Source: CAD feature listing. Evaluate the final solid. Frame: model axes, mm. Face numbers are marked on the shaded views. A direction names the side the tool comes from. Give positions to 0.01 mm unless a question says otherwise; leave off trailing zeros. Order: outer loops, then holes, each group sorted by start corner. A loop starts at its lowest first (then second) coordinate and runs counter-clockwise, first axis right, second up.
```python
from build123d import *

# Parameters (mm, degrees)
SKETCH1_R           = 1.6
BOSS_EXTRUDE1_DEPTH = 10
CAVITY1_OUTLINE_R   = 1.25
CAVITY1_DEPTH       = 6.34
CAVITY1_START       = -22.606898648
CAVITY1_2_OUTLINE_R = 0.9
CAVITY1_2_DEPTH     = 0.47
CAVITY1_START_2     = -15.306898648
CAVITY1_3_OUTLINE_R = 0.9
CAVITY1_3_DEPTH     = 0.47
CAVITY1_START_3     = -6.506898648
CAVITY1_4_OUTLINE_R = 0.9
CAVITY1_4_DEPTH     = 0.47
CUT_EXTRUDE2_REACH  = 54.912
SKETCH2_R           = 1.15
CUT_EXTRUDE3_START  = -3.5
SKETCH3_R           = 1.15
CUT_EXTRUDE3_DEPTH  = 3.5
FILLET1_R           = 1
FILLET2_R           = 5
CUT_EXTRUDE4_START  = -6.34
CUT_EXTRUDE4_DEPTH  = 6.34
FILLET3_R           = 2
FILLET4_R           = 2
FILLET5_R           = 0.5


with BuildPart() as part:
    # Sketch1 → Boss-Extrude1 (new body)
    with BuildSketch(Plane.XY):
        Polygon((0, 0), (25.6, 0), (38.35, -30.037117664), (38.35, -35.9), (15.869351212, -35.9), (0, -28.5), align=None)
        with Locations((31.648794461, -31.570900751)):
            Circle(SKETCH1_R, mode=Mode.SUBTRACT)
        with Locations((21.498394042, -9.298229799)):
            Circle(SKETCH1_R, mode=Mode.SUBTRACT)
    extrude(amount=BOSS_EXTRUDE1_DEPTH)

    # Cavity1: read off the stored shape, not the designer's step
    # Cavity1 outline → Cavity1 (cut)
    with BuildSketch(Plane.XY):
        Polygon((10.198394042, -24.671898648), (10.198394042, -21.671898648), (10.808394042, -21.171898648), (10.808394042, -18.171898648), (10.198394042, -17.671898648), (10.198394042, -12.171898648), (10.808394042, -11.671898648), (10.808394042, -8.671898648), (10.198394042, -8.171898648), (10.198394042, -4.671898648), (0, -4.671898648), (0, -14.603899938), (0.718394042, -15.191898648), (0.718394042, -24.671898648), align=None)
        with Locations((7.908394042, -19.671898648)):
            Circle(CAVITY1_OUTLINE_R, mode=Mode.SUBTRACT)
        with Locations((7.908394042, -10.171898648)):
            Circle(CAVITY1_OUTLINE_R, mode=Mode.SUBTRACT)
    extrude(amount=CAVITY1_DEPTH, mode=Mode.SUBTRACT)

    # Cavity1 2 outline → Cavity1 2 (cut)
    with BuildSketch(Plane(origin=(0, 0, 0), x_dir=(1, 0, 0), z_dir=(0, 1, 0)).offset(CAVITY1_START)):
        Polygon((13.478394042, -4.73), (14.198394042, -4.01), (14.198394042, -2.33), (13.478394042, -1.61), (10.198394042, -1.61), (10.198394042, -4.73), align=None)
        with Locations((12.398394042, -3.17)):
            Circle(CAVITY1_2_OUTLINE_R, mode=Mode.SUBTRACT)
    extrude(amount=CAVITY1_2_DEPTH, mode=Mode.SUBTRACT)

    # Cavity1 3 outline → Cavity1 3 (cut)
    with BuildSketch(Plane(origin=(0, 0, 0), x_dir=(1, 0, 0), z_dir=(0, 1, 0)).offset(CAVITY1_START_2)):
        Polygon((13.478394042, -4.73), (14.198394042, -4.01), (14.198394042, -2.33), (13.478394042, -1.61), (10.198394042, -1.61), (10.198394042, -4.73), align=None)
        with Locations((12.398394042, -3.17)):
            Circle(CAVITY1_3_OUTLINE_R, mode=Mode.SUBTRACT)
    extrude(amount=CAVITY1_3_DEPTH, mode=Mode.SUBTRACT)

    # Cavity1 4 outline → Cavity1 4 (cut)
    with BuildSketch(Plane(origin=(0, 0, 0), x_dir=(1, 0, 0), z_dir=(0, 1, 0)).offset(CAVITY1_START_3)):
        Polygon((13.478394042, -4.73), (14.198394042, -4.01), (14.198394042, -2.33), (13.478394042, -1.61), (10.198394042, -1.61), (10.198394042, -4.73), align=None)
        with Locations((12.398394042, -3.17)):
            Circle(CAVITY1_4_OUTLINE_R, mode=Mode.SUBTRACT)
    extrude(amount=CAVITY1_4_DEPTH, mode=Mode.SUBTRACT)

    # Cut-Extrude2: up to this face of the body (flat: up to its plane)
    cut_extrude2_end = Plane(part.part.faces().sort_by_distance((19.850612991, -19.341556746, 0))[0])
    # Sketch2 → Cut-Extrude2 (cut, up to the picked face)
    with BuildSketch(Plane(origin=(0, 0, 6.34), x_dir=(-1, 0, 0), z_dir=(0, 0, -1)), mode=Mode.PRIVATE) as cut_extrude2_sk1:
        Polygon((-10.908394042, -21.219231953), (-10.298394042, -21.719231953), (-10.298394042, -24.771898648), (-0.618394042, -24.771898648), (-0.618394042, -15.239275241), (0.1, -14.651276531), (0.1, -4.571898648), (-10.298394042, -4.571898648), (-10.298394042, -8.124565343), (-10.908394042, -8.624565343), (-10.908394042, -11.719231953), (-10.298394042, -12.219231953), (-10.298394042, -17.624565343), (-10.908394042, -18.124565343), align=None)
        with Locations((-7.908394042, -10.171898648)):
            Circle(SKETCH2_R, mode=Mode.SUBTRACT)
        with Locations((-7.908394042, -19.671898648)):
            Circle(SKETCH2_R, mode=Mode.SUBTRACT)
    cut_extrude2_tool1 = split(extrude(cut_extrude2_sk1.sketch, amount=CUT_EXTRUDE2_REACH, mode=Mode.PRIVATE), bisect_by=cut_extrude2_end, keep=Keep.BOTH, mode=Mode.PRIVATE)
    add(cut_extrude2_tool1.solids().sort_by(Axis((5.274649, -14.483088, 6.34), (0, 0, -1)))[0], mode=Mode.SUBTRACT)

    # Sketch3 → Cut-Extrude3 (cut)
    with BuildSketch(Plane(origin=(0, 0, 0), x_dir=(-1, 0, 0), z_dir=(0, 0, -1)).offset(CUT_EXTRUDE3_START)):
        with Locations((-7.908394042, -10.171898648)):
            Circle(SKETCH3_R)
        with Locations((-7.908394042, -19.671898648)):
            Circle(SKETCH3_R)
    extrude(amount=CUT_EXTRUDE3_DEPTH, mode=Mode.SUBTRACT)

    # Fillet1
    fillet1_edges = [part.edges().sort_by_distance(p)[0] for p in [
        (9.058394042, -10.171898648, 3.5),
        (9.058394042, -19.671898648, 3.5),
    ]]
    fillet(fillet1_edges, radius=FILLET1_R)

    # Fillet2
    fillet2_edges = [part.edges().sort_by_distance(p)[0] for p in [
        (25.6, 0, 5),
        (38.35, -30.037117664, 5),
    ]]
    fillet(fillet2_edges, radius=FILLET2_R)

    # Sketch4 → Cut-Extrude4 (cut)
    with BuildSketch(Plane(origin=(0, 0, 0), x_dir=(-1, 0, 0), z_dir=(0, 0, -1)).offset(CUT_EXTRUDE4_START)):
        Polygon((-10.298394042, -5.850997484), (-15.298394042, -5.850997484), (-23.35, -35.9), (-17.655981008, -35.9), (-14.377222224, -23.663505632), (-10.298394042, -23.663505632), (-10.298394042, -21.719231953), (-13.908394042, -21.719231953), (-13.908394042, -16.124565343), (-10.298394042, -16.124565343), (-10.298394042, -14.124565343), (-13.908394042, -14.124565343), (-13.908394042, -7.374565343), (-10.298394042, -7.374565343), align=None)
    extrude(amount=CUT_EXTRUDE4_DEPTH, mode=Mode.SUBTRACT)

    # Fillet3
    fillet3_edges = [part.edges().sort_by_distance(p)[0] for p in [
        (14.377222224, -23.663505632, 3.17),
        (13.908394042, -21.719231953, 3.17),
        (13.908394042, -16.124565343, 3.17),
        (13.908394042, -14.124565343, 3.17),
        (13.908394042, -7.374565343, 3.17),
    ]]
    fillet(fillet3_edges, radius=FILLET3_R)

    # Fillet4
    fillet4_edges = [part.edges().sort_by_distance(p)[0] for p in [
        (15.298394042, -5.850997484, 3.17),
    ]]
    fillet(fillet4_edges, radius=FILLET4_R)

    # Fillet5
    fillet5_edges = [part.edges().sort_by_distance(p)[0] for p in [
        (10.298394042, -5.850997484, 3.17),
        (10.298394042, -23.663505632, 3.17),
    ]]
    fillet(fillet5_edges, radius=FILLET5_R)


solid = part.part
```
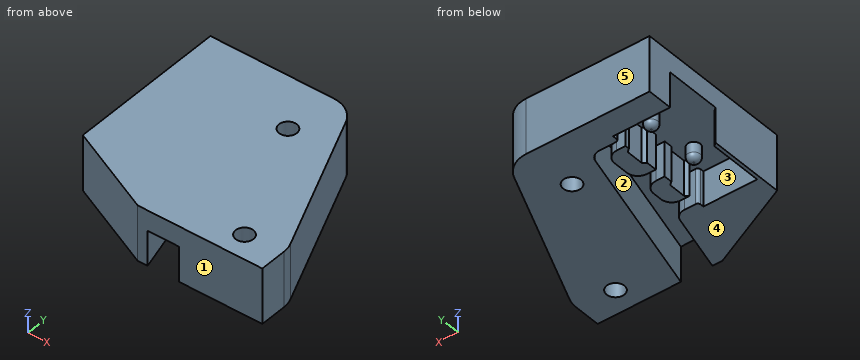
1) Pin query (flat end, axial travel): pin 1 (1.3 mm diameter, centred on x = 11, z = 3.5, fed in from -Y); pin 2 (0.5 mm diameter, centred on y = -19, z = 2.5, fed in from +X); pin 3 (1.5 mm diameter, centred on x = 27.5, z = 2, fed in from +Y); pin 4 (2.5 mm diameter, centred on x = 31.65, y = -31.57, fed in from -Z) (3 decimals). Return the tip coordinate at first contact, or that it passes through.
Report:
pin 1: stops at y = -33.93
pin 2: stops at x = 33.77
pin 3: stops at y = -2.74
pin 4: passes through
2) Section query B-B, the plane z = 7. Return the cut outline in (x, y), and give its area (3 significant figures).
Report:
outline: (0, -28.5) - (15.87, -35.9) - (38.35, -35.9) - (38.35, -31.05) arc R5 ccw to (37.95, -29.1) - (26.89, -3.05) arc R5 ccw to (22.29, 0) - (0, 0) - close; hole circle Ø3.2 at (21.5, -9.3); hole circle Ø3.2 at (31.65, -31.57)
area: 1,110 mm2
3) Section query A-A, the plane x = 32.5. Return the cut outline in (y, z).
Report:
outline: (-35.9, 0) - (-32.93, 0) - (-32.93, 10) - (-35.9, 10) - close; (-30.22, 0) - (-16.26, 0) - (-16.26, 10) - (-30.22, 10) - close
4) Section query C-C, the plane x = 4. Return the cut outline in (y, z), and give its area (3 significant figures).
Report:
outline: (-30.37, 0) - (-24.77, 0) - (-24.77, 6.34) - (-4.57, 6.34) - (-4.57, 0) - (0, 0) - (0, 10) - (-30.37, 10) - close
area: 176 mm2
5) Material intervals for L1, parallel to Z at x = 13, y = -6.5; L2, parallel to X at y = -9, z = 2; L3, parallel to X at y = -20.5, z = 3.5, sorted ascending.
Report:
L1: z = 6.34 to 10
L2: x = 10.91 to 13.87, 16.14 to 19.93, 23.07 to 29.42
L3: x = 0 to 0.62, 10.91 to 13.75, 19.22 to 34.3
6) Section query D-D, the plane z = 2.75. Count the separate pieces of the cut face and the enclosed holes in it, and give its area (3 significant figures).
Report:
separate pieces: 4
enclosed holes: 2
area: 742 mm2
7) Reachability of the marked faces 1 and 2 from +Z, -Z, +X, -X, +Y, -Y: full face, straight path, thin tool, end or side. Return the list, or none.
Report:
face 1: +Z, -Z, +X, -X, -Y
face 2: -Z
8) Draft query along Y for the marked faces 3, 4 and 5. Return one class per face: +Y half, -Y half, draft (parallel to the pull), parting line (faces both ways), or undercut.
Report:
face 3: undercut
face 4: draft
face 5: +Y half
